Verification items for the finished model (mm, model axes). Coordinates: 2 decimals unless noted, no trailing zeros. Order: outer loops, then holes, each group sorted by start corner. A loop starts at its lowest first (then second) coordinate and runs counter-clockwise, first axis right, second up. Notation, with made-up numbers: M -15.5,13 L 24.5,13 A18 ccw 24.5,27 Z; hole C 13,72.5 d8. An arc over 180 degrees is marked long. Return JSON: item names as keys, results as strings. Group by question number.
Q1. Section check D-D, the plane z = 6. Enter the section's corners in (x, y), then the cut area to 3 significant figures.
Q2. Section check C-C, the plane z = 25. Enter the section's corners in (x, y).
Q3. Section check B-B, the plane x = -24. Enter the section's corners in (y, z), then the cut area to 3 significant figures.
Q4. Thickness scan on probe 1 along X at (y, z) = (55.5, 13); probe 2 along X at (y, z) = (-122.5, 23.5); probe 3 along Y at (x, z) = (76, 13). Record the ranges inside material, lowest first.
Q5. Go/stop test with flat-tipped pins: pin 1 Ø3 at (y, z) = (101, 29) entering from -X; pin 2 Ø8 at (x, z) = (142, 8.5) entering from -Y; pin 3 Ø1 at (x, z) = (31, 25.5) entering from +Y; pin 4 Ø6 at (y, z) = (-34.5, 7.5) entering from +X. Record where each tip stops, or that it passes through.
Q6. Section check A-A, the plane y = 90.5. Enter the section's corners in (x, z).
from build123d import *

# Parameters (mm, degrees)
F0_W     = 410
F0_H     = 310
F1_DEPTH = 35
F3_DEPTH = 413
F7_DEPTH = 455


with BuildPart() as f1:
    # F0 (on Top) → F1 (new body)
    with BuildSketch(Plane.XY):
        Rectangle(F0_W, F0_H)
    extrude(amount=F1_DEPTH)


with BuildPart() as f3:
    # F2 (on face) → F3 (new body)
    with BuildSketch(Plane.XZ.offset(155)):
        Polygon((-186.286226, -45.123053), (-145, 0), (-205, 30), (-247.468904, 11.412853), align=None)
    extrude(amount=-F3_DEPTH)


with BuildPart() as f4_1:
    # F4: instance of F3
    add(f3.part.mirror(Plane.YZ))


with BuildPart() as f1_1:
    add(f1.part)

    # F5: cut F3, F4_1
    add(f3.part, mode=Mode.SUBTRACT)
    add(f4_1.part, mode=Mode.SUBTRACT)


with BuildPart() as f7:
    # F6 (on face) → F7 (new body)
    with BuildSketch(Plane(origin=(-205, 0, 0), x_dir=(0, -1, 0), z_dir=(-1, 0, 0))):
        Polygon((-155, -27.468236), (-95, 0), (-155, 30), (-189.205855, 15.520646), align=None)
    extrude(amount=-F7_DEPTH)


with BuildPart() as f8_1:
    # F8: instance of F7
    add(f7.part.mirror(Plane.XZ))


with BuildPart() as f1_2:
    add(f1_1.part)

    # F9: cut F7, F8_1
    add(f7.part, mode=Mode.SUBTRACT)
    add(f8_1.part, mode=Mode.SUBTRACT)


solid = f1_2.part
Numbers:
{
 "1": {"outline": "M -157,-107 L 157,-107 L 157,107 L -157,107 Z", "area": "67,200 mm2"},
 "2": {"outline": "M -195,-145 L 195,-145 L 195,145 L -195,145 Z"},
 "3": {"outline": "M -155,30 L -95,0 L 95,0 L 155,30 L 155,35 L -155,35 Z", "area": "9,050 mm2"},
 "4": {"probe 1": "x = -171 to 171", "probe 2": "x = -192 to 192", "probe 3": "y = -121 to 121"},
 "5": {"pin 1": "stops at x = -205", "pin 2": "stops at y = -120", "pin 3": "stops at y = 147", "pin 4": "stops at x = 166"},
 "6": {"outline": "M -205,30 L -145,0 L 145,0 L 205,30 L 205,35 L -205,35 Z"}
}
